```python
from build123d import *

# Parameters (mm, degrees)
F1_DEPTH = 25.4
F2_DEPTH = 38.1


with BuildPart() as f1:
    # F0 (on Top) → F1 (new body)
    with BuildSketch(Plane.XY):
        with BuildLine():
            Line((49.0129638637, 29.9626197666), (46.774469316, 29.9626197666))
            ThreePointArc((46.774469316, 29.9626197666), (30.3001427561, 29.390654175), (13.8258161962, 29.9626197666))
            Line((13.8258161962, 29.9626197666), (-21.1371275652, 29.9626197666))
            ThreePointArc((-21.1371275652, 29.9626197666), (-11.4921190987, 16.3403500801), (-8.0883889408, 0))
            ThreePointArc((-8.0883889408, 0), (-11.4921190987, -16.3403500801), (-21.1371275652, -29.9626197666))
            Line((-21.1371275652, -29.9626197666), (49.0129638637, -29.9626197666))
            Line((49.0129638637, -29.9626197666), (49.0129638637, 29.9626197666))
        make_face()
        with BuildLine():
            Line((-49.0129638637, 29.9626197666), (-21.1371275652, 29.9626197666))
            ThreePointArc((-21.1371275652, 29.9626197666), (-28.7111277901, 35.5338751709), (-37.3567476866, 39.2294972827))
            ThreePointArc((-37.3567476866, 39.2294972827), (-88.8574497894, -9.3401163775), (-21.1371275652, -29.9626197666))
            Line((-21.1371275652, -29.9626197666), (-49.0129638637, -29.9626197666))
            Line((-49.0129638637, -29.9626197666), (-49.0129638637, -29.141463528))
            ThreePointArc((-49.0129638637, -29.141463528), (-78.1544273918, 0), (-49.0129638637, 29.141463528))
            Line((-49.0129638637, 29.141463528), (-49.0129638637, 29.9626197666))
        make_face()
        with BuildLine():
            ThreePointArc((-8.0883889408, 0), (-11.4921190987, 16.3403500801), (-21.1371275652, 29.9626197666))
            Line((-21.1371275652, 29.9626197666), (-49.0129638637, 29.9626197666))
            Line((-49.0129638637, 29.9626197666), (-49.0129638637, 29.141463528))
            ThreePointArc((-49.0129638637, 29.141463528), (-28.4068373894, 20.6061264744), (-19.8715003357, 0))
            ThreePointArc((-19.8715003357, 0), (-28.4068373894, -20.6061264744), (-49.0129638637, -29.141463528))
            Line((-49.0129638637, -29.141463528), (-49.0129638637, -29.9626197666))
            Line((-49.0129638637, -29.9626197666), (-21.1371275652, -29.9626197666))
            ThreePointArc((-21.1371275652, -29.9626197666), (-11.4921190987, -16.3403500801), (-8.0883889408, 0))
        make_face()
    extrude(amount=F1_DEPTH)

    # F0 (on Top) → F2 (join)
    with BuildSketch(Plane.XY):
        with BuildLine():
            ThreePointArc((-19.8715003357, 0), (-28.4068373894, 20.6061264744), (-49.0129638637, 29.141463528))
            Line((-49.0129638637, 29.141463528), (-49.0129638637, 22.6363457986))
            ThreePointArc((-49.0129638637, 22.6363457986), (-33.0066502483, 16.0063136155), (-26.3766180651, 0))
            ThreePointArc((-26.3766180651, 0), (-33.0066502483, -16.0063136155), (-49.0129638637, -22.6363457986))
            Line((-49.0129638637, -22.6363457986), (-49.0129638637, -29.141463528))
            ThreePointArc((-49.0129638637, -29.141463528), (-28.4068373894, -20.6061264744), (-19.8715003357, 0))
        make_face()
        with BuildLine():
            Line((-49.0129638637, 22.6363457986), (-49.0129638637, 29.141463528))
            ThreePointArc((-49.0129638637, 29.141463528), (-78.1544273918, 0), (-49.0129638637, -29.141463528))
            Line((-49.0129638637, -29.141463528), (-49.0129638637, -22.6363457986))
            ThreePointArc((-49.0129638637, -22.6363457986), (-71.6493096624, 0), (-49.0129638637, 22.6363457986))
        make_face()
    extrude(amount=F2_DEPTH)


solid = f1.part
```
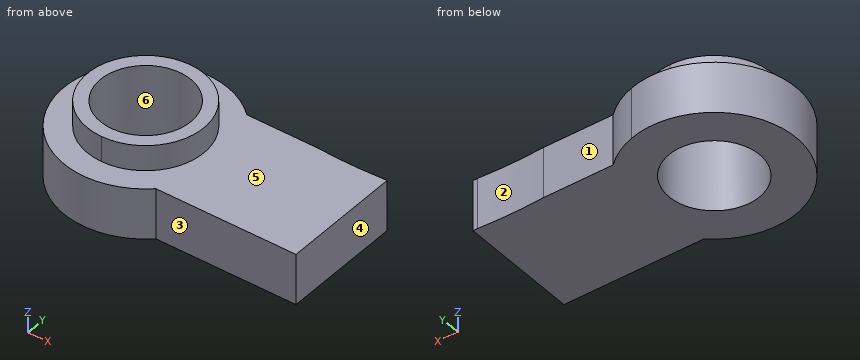
Can you work these out from the model? Positions are in its coordinate system, mm. Face numbers are marked on the shaded views. A direction names the side the tool comes from. Round coordinates to 2 decimals unless told otherwise and drop trailing zeros. Order: outer loops, then holes, each group sorted by start corner. A loop starts at its lowest first (then second) coordinate and runs counter-clockwise, first axis right, second up.
(1) If we section it at B-B (z = 9): Please give me the cut outline in (x, y).
Results are:
outline: (-21.14, -29.96) - (49.01, -29.96) - (49.01, 29.96) - (46.77, 29.96) arc R237.54 cw to (13.83, 29.96) - (-21.14, 29.96) arc R40.92 ccw (long way) to start; hole circle Ø45.27 at (-49.01, 0)
(2) If I drill on L1, parallel to Y at x = 3, z = 23; L2, parallel to Y at x = 29.5, z = 14; L3, parallel to Y at x = -50, z = 32, over which ranges is the centre line in solid material (lowest first)?
Results are:
L1: y = -29.96 to 29.96
L2: y = -29.96 to 29.39
L3: y = -29.12 to -22.61, 22.61 to 29.12
(3) On a 3-axis mill with a long thin cutter (end or side, diameter ignored), from which of +Z, -Z, +X, -X, +Y, -Y can I reach the whole of each face in a straight line? I mean the marked faces 1, 2 and 3. Say none if no direction works.
Results are:
face 1: +Z, -Z, +X, +Y
face 2: +Z, -Z, +Y
face 3: +Z, -Z, +X, -Y
(4) If we section it at A-A (y = 0): Please give me the cut outline in (x, z), plus the area to 3 significant figures.
Results are:
outline: (-89.94, 0) - (-71.65, 0) - (-71.65, 38.1) - (-78.15, 38.1) - (-78.15, 25.4) - (-89.94, 25.4) - close; (-26.38, 0) - (49.01, 0) - (49.01, 25.4) - (-19.87, 25.4) - (-19.87, 38.1) - (-26.38, 38.1) - close
area: 2,540 mm2
(5) If we section it at D-D (x = -2.5): Please give me the cut outline in (y, z).
Results are:
outline: (-29.96, 0) - (29.96, 0) - (29.96, 25.4) - (-29.96, 25.4) - close
(6) I'm going to push flat-ended pins straight in: pin 1 (8 mm diameter, centred on x = 23.5, y = 28.5, fed in from +Z); pin 2 (8 mm diameter, centred on x = -31.5, z = 18.5, fed in from +Y); pin 3 (6 mm diameter, centred on x = -76, z = 32.5, fed in from -Y). Where does each tip first touch, or does it pass through?
Results are:
pin 1: stops at z = 25.4
pin 2: stops at y = 38.63
pin 3: stops at y = -16.55
(7) We'd pull the mould along X, two halves only. Please class the marked faces 4, 5 and 6: +X half, -X half, draft (parallel to the pull), parting line (faces both ways), or undercut.
Results are:
face 4: +X half
face 5: draft
face 6: undercut
(8) If we section it at C-C (x = -59.5): Please give me the cut outline in (y, z), plus the area to 3 significant figures.
Results are:
outline: (-39.56, 0) - (-20.06, 0) - (-20.06, 38.1) - (-27.19, 38.1) - (-27.19, 25.4) - (-39.56, 25.4) - close; (20.06, 0) - (39.56, 0) - (39.56, 25.4) - (27.19, 25.4) - (27.19, 38.1) - (20.06, 38.1) - close
area: 1,170 mm2
